Part model, mm, in its own coordinate system. Face numbers are marked on the shaded views. A direction names the side the tool comes from. Round coordinates to 2 decimals unless told otherwise and drop trailing zeros. Order: outer loops, then holes, each group sorted by start corner. A loop starts at its lowest first (then second) coordinate and runs counter-clockwise, first axis right, second up. Notation, with made-up numbers: (-2.5, 57) - (38.5, 57) arc R23 ccw to (38.5, 83) - close; hole circle Ø8 at (21, -26.75). An arc over 180 degrees is marked (long way). Return JSON: item names as keys, results as strings. Group by question number.
Item 1: Saw through at D-D on z = 164.5. List the corners of the cut face in (x, y), and give its area (3 significant figures).
Item 2: Drop flat-ended pins along their axis: pin 1 (3 mm diameter, centred on x = 73.5, y = -91, fed in from -Z); pin 2 (8 mm diameter, centred on y = -166, z = 183.5, fed in from -X); pin 3 (8 mm diameter, centred on x = 37.18, y = -190, fed in from +Z); pin 4 (5.5 mm diameter, centred on x = 37.18, y = -10, fed in from +Z). Give the stop position or say it passes through.
Item 3: Tool access for the marked faces 1, 2 and 3: list every direction of +Z, -Z, +X, -X, +Y, -Y with a clear straight run to the whole face (end or side of a thin tool).
Item 4: Saw through at B-B on x = 54. List the corners of the cut face in (y, z), and give its area (3 significant figures).
Item 5: Probe probe 1 along Z at (x, y) = (47, -33.5); probe 2 along Z at (x, y) = (257.5, -173); probe 3 along X at (y, z) = (-110, 130.5). List the from-to ranges inside material, lowest first.
Solid Edge part; units mm, degrees
sketch "Sketch1" plane through (0, 0, 0) normal (0, -1, 0) x (1, 0, 0)
  line L0 (77.3764, 199.2749) -> (17.3764, 199.2749)
  line L1 (17.3764, 199.2749) -> (17.3764, 196.2749)
  line L2 (17.3764, 196.2749) -> (77.3764, 196.2749)
  arc A0 (77.3764, 196.2749) -> (128.9473, 155.7325) centre (83.2091, 150.6232) cw
  arc A1 (128.9473, 155.7325) -> (179.9264, 103.2749) centre (179.9264, 154.2749) ccw
  line L3 (269.9264, 103.2749) -> (179.9264, 103.2749)
  line L4 (269.9264, 106.2749) -> (269.9264, 103.2749)
  line L5 (179.9264, 106.2749) -> (269.9264, 106.2749)
  arc A2 (131.9471, 155.6831) -> (179.9264, 106.2749) centre (179.9264, 154.2749) ccw
  arc A3 (77.3764, 199.2749) -> (131.9471, 155.6831) centre (83.2091, 150.6232) cw
  dimension "D1" = 17.3764
  dimension "D2" = 77.3764
  dimension "D3" = 179.9264
  dimension "D4" = 269.9264
  dimension "D5" = 269.9264
extrude "Protrusion1" add sketch "Sketch1" along normal blind 200
fillet "Verrundung_4" radius 3 1 edges at (269.9264, -100, 106.2749)
sketch "Sketch2" plane through (223.4264, -100, 106.2749) normal (0, 0, 1) x (1, 0, 0)
  circle A0 centre (-13.5, 40) radius 3.5
  circle A1 centre (-13.5, -40) radius 3.5
  dimension "D1" = 13.5
extrude "Cutout1" cut sketch "Sketch2" against normal through all
sketch "Sketch3" plane through (143.6514, -200, 152.9362) normal (0, -1, 0) x (1, 0, 0)
  line L0 (-126.275, 37.3386) -> (-126.275, 43.3386)
  line L1 (-126.275, 43.3386) -> (-126.275, 46.3386)
  line L2 (-126.275, 46.3386) -> (-66.275, 46.3386)
  line L3 (-66.275, 46.3386) -> (-50.0814, 44.2327)
  line L4 (-50.0814, 44.2327) -> (-37.0073, 38.973)
  line L5 (-37.0073, 38.973) -> (-35.5454, 37.3386)
  line L6 (-35.5454, 37.3386) -> (-126.275, 37.3386)
extrude "Protrusion2" add sketch "Sketch3" against normal up to vertex (200 mm away)
sketch "Sketch4" plane through (47.3764, -100, 199.2749) normal (0, 0, 1) x (1, 0, 0)
  circle A0 centre (-10.2, 90) radius 3.5
  circle A1 centre (-10.2, -90) radius 3.5
  dimension "D1" = 10.2
  dimension "D2" = 10.2
  dimension "D3" = 10.2
extrude "Cutout2" cut sketch "Sketch4" against normal through all
sketch "Sketch5" plane through (143.6514, -200, 151.449) normal (0, -1, 0) x (1, 0, 0)
  line L0 (-126.275, 47.8258) -> (-66.275, 47.8258)
  line L1 (-66.275, 47.8258) -> (-66.275, 41.8258)
  line L2 (-66.275, 41.8258) -> (-126.275, 41.8258)
  line L3 (-126.275, 41.8258) -> (-126.275, 47.8258)
extrude "Cutout3" cut sketch "Sketch5" against normal through all
properties material "Nylon, allgemein"
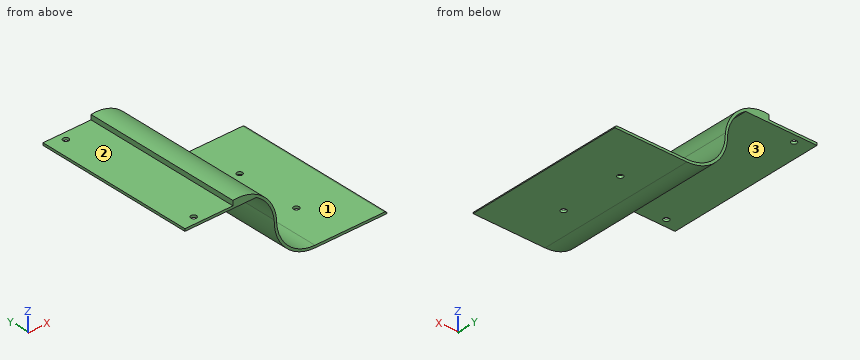
Filled in:
{
 "1": {"outline": "(127.09, -200) - (130.2, -200) - (130.2, 0) - (127.09, 0) - close", "area": "623 mm^2"},
 "2": {"pin 1": "stops at z = 190.27", "pin 2": "stops at x = 110.74", "pin 3": "stops at z = 193.27", "pin 4": "passes through"},
 "3": {"face 1": "+Z, +X, +Y, -Y", "face 2": "+Z, -X, +Y, -Y", "face 3": "-Z, -X, +Y, -Y"},
 "4": {"outline": "(-200, 190.27) - (0, 190.27) - (0, 193.27) - (-200, 193.27) - close", "area": "600 mm^2"},
 "5": {"probe 1": "z = 190.27 to 193.27", "probe 2": "z = 103.27 to 106.27", "probe 3": "x = 134.81 to 138.23"}
}
